Geometry check sheet. Reference: the model listing, model coordinates, mm. A direction names the side the tool comes from. Coordinates: 2 decimals unless noted, no trailing zeros. Write each loop counter-clockwise with the first axis right and the second up, starting at its lowest first coordinate (ties: lowest second). Pieces come first, ordered by that corner, then holes. Notation, with made-up numbers: (64, 69) -> (111, 69) arc R31 cw to (111, 107) -> close; hole circle Ø8 at (19.25, -14.75). An arc over 180 degrees is marked (long way). Put each result on its own line as item: value. Start each with the question number.
from build123d import *

# Parameters (mm, degrees)
EXTRUDE_1_DEPTH     = 40
SKETCH_4_W          = 8
SKETCH_4_H          = 8
EXTRUDE_2_DEPTH     = 8
SKETCH_5_R          = 1.98
CUT_EXTRUDE_2_DEPTH = 8
FILLET_1_R          = 10
FILLET_2_R          = 10
SKETCH_6_W          = 8
SKETCH_6_H          = 8
EXTRUDE_3_DEPTH     = 8
SKETCH_7_R          = 1.98
CUT_EXTRUDE_3_DEPTH = 8
FILLET_3_R          = 10
FILLET_4_R          = 10


with BuildPart() as part:
    # 草图2 → 凸台-拉伸1 (new body)
    with BuildSketch(Plane(origin=(0, 0, 0), x_dir=(0, 0, -1), z_dir=(1, 0, 0))):
        Polygon((0, 0), (0, -42), (-25.455844123, -67.455844123), (-27.930717857, -64.980970389), (-3.5, -40.550252532), (-3.5, 0), align=None)
    extrude(amount=EXTRUDE_1_DEPTH)

    # 草图4 → 凸台-拉伸2 (add)
    with BuildSketch(Plane.ZY):
        with Locations((1.75, -4)):
            Rectangle(SKETCH_4_W, SKETCH_4_H)
    extrude(amount=EXTRUDE_2_DEPTH)

    # 草图5 → 切除-拉伸2 (cut)
    with BuildSketch(Plane(origin=(0, 0, 0), x_dir=(1, 0, 0), z_dir=(0, 1, 0))):
        with Locations(Location((-4, -1.75, 0), (0, 0, 270))):
            Circle(SKETCH_5_R)
    extrude(amount=-CUT_EXTRUDE_2_DEPTH, mode=Mode.SUBTRACT)

    # 圆角1
    # the kernel refuses this fillet: 10 mm, written as the material it adds along each edge
    with BuildSketch(Plane(origin=(0, 0, 0), x_dir=(1, 0, 0), z_dir=(0, -1, 0))) as fillet_1_piece_1:
        with BuildLine():
            CenterArc((6.31961233, -10), FILLET_1_R, 90, 39.194967426)
            Line((0, -2.25), (0, 0))
            Line((0, 0), (6.31961233, 0))
        make_face()
    extrude(amount=8)

    # 圆角2
    # the kernel refuses this fillet: 10 mm, written as the material it adds along each edge
    with BuildSketch(Plane(origin=(0, -8, 3.5), x_dir=(1, 0, 0), z_dir=(0, 1, 0))) as fillet_2_piece_1:
        with BuildLine():
            CenterArc((6.31961233, -10), FILLET_2_R, 90, 39.194967426)
            Line((0, -2.25), (0, 0))
            Line((0, 0), (6.31961233, 0))
        make_face()
    extrude(amount=8)

    # 草图6 → 凸台-拉伸3 (add)
    with BuildSketch(Plane(origin=(40, 0, 0), x_dir=(0, 0, -1), z_dir=(1, 0, 0))):
        with Locations((-1.75, -4)):
            Rectangle(SKETCH_6_W, SKETCH_6_H)
    extrude(amount=EXTRUDE_3_DEPTH)

    # 草图7 → 切除-拉伸3 (cut)
    with BuildSketch(Plane(origin=(0, 0, 0), x_dir=(1, 0, 0), z_dir=(0, 1, 0))):
        with Locations(Location((44, -1.75, 0), (0, 0, 270))):
            Circle(SKETCH_7_R)
    extrude(amount=-CUT_EXTRUDE_3_DEPTH, mode=Mode.SUBTRACT)

    # 圆角3
    # the kernel refuses this fillet: 10 mm, written as the material it adds along each edge
    with BuildSketch(Plane(origin=(40, 0, 0), x_dir=(-1, 0, 0), z_dir=(0, -1, 0))) as fillet_3_piece_1:
        with BuildLine():
            CenterArc((6.31961233, 10), FILLET_3_R, 230.805032574, 39.194967426)
            Line((0, 2.25), (0, 0))
            Line((0, 0), (6.31961233, 0))
        make_face()
    extrude(amount=8)

    # 圆角4
    # the kernel refuses this fillet: 10 mm, written as the material it adds along each edge
    with BuildSketch(Plane(origin=(40, -8, 3.5), x_dir=(-1, 0, 0), z_dir=(0, 1, 0))) as fillet_4_piece_1:
        with BuildLine():
            CenterArc((6.31961233, 10), FILLET_4_R, 230.805032574, 39.194967426)
            Line((0, 2.25), (0, 0))
            Line((0, 0), (6.31961233, 0))
        make_face()
    extrude(amount=8)


solid = part.part
Item 1: Section check C-C, the plane y = -31. Enter the section's corners in (x, z), and give its area (3 significant figures).
Item 2: Section check D-D, the plane x = 21.5. Enter the section's corners in (y, z), and give its area (3 significant figures).
Item 3: Scan lines: line 1 along X through (y, z) = (-3.75, 1.75); line 2 along Z through (x, y) = (6, -31); line 3 along Y through (x, z) = (-1.5, 5). Record each from-to range of solid material in increasing order. Write a range as [from, to].
Item 4: Section check A-A, the plane z = 1.75. Enter the section's corners in (x, y), and give its area (3 significant figures).
Item 5: Access from +Z, -Z, +X, -X, +Y, -Y to the whole of each face (thin tool, end or side, straight path). Record for faces 1 (the flat face through (20, -21, 0)), 2 (the flat face through (20, -21, 3.5)), 3 (the cylindrical face through (37.08, -3.944, -0.595)), 4 (the flat face through (0, -42, 4.6)), 5 (the cylindrical face through (3.011, -4.056, 4.063)).
Item 6: Mould release check, pull along Z, two halves, no side actions. Record for faces 6 (the cylindrical face through (45.963, -3.944, 1.492)), 7 (the flat face through (19.72, -66.236, 26.676)), 8 (the flat face through (40, -42, 4.6)): released by +Z, released by -Z, zero draft, split by the parting line, or undercut.
Item 7: Go/stop test with flat-tipped pins: P1, Ø12, axis at x = 26.5, y = -28, coming from the -Z side; P2, Ø1.5, axis at x = 5, y = -53, coming from the -Z side; P3, Ø10, axis at x = -1, y = -10, coming from the +Z side; P4, Ø8.5, axis at y = -26, z = 9, coming from the -X side. Record where each tip stops, or that it passes through.
Item 8: Section check B-B, the plane x = -4. Enter the section's corners in (y, z).
From the geometry:
1. outline: (0, 0) -> (40, 0) -> (40, 3.5) -> (0, 3.5) -> close
1. area: 140 mm²
2. outline: (-67.46, 25.46) -> (-42, 0) -> (0, 0) -> (0, 3.5) -> (-40.55, 3.5) -> (-64.98, 27.93) -> close
2. area: 268 mm²
3. line 1: [-8, -5.98], [-2.02, 42.02], [45.98, 48]
3. line 2: [0, 3.5]
3. line 3: [-8, 0]
4. outline: (-8, -8) -> (-5.98, -8) -> (-5.98, 0) -> (-8, 0) -> close; (-2.02, -8) -> (0, -8) -> (0, -43.75) -> (40, -43.75) -> (40, -8) -> (42.02, -8) -> (42.02, 0) -> (-2.02, 0) -> close; (45.98, -8) -> (48, -8) -> (48, 0) -> (45.98, 0) -> close
4. area: 1,810 mm²
5. face 1: -Z, -Y
5. face 2: +Z
5. face 3: -Z, +Y, -Y
5. face 4: +Z, -Z, -X, -Y
5. face 5: +Z, +Y
6. face 6: undercut
6. face 7: released by +Z
6. face 8: zero draft
7. P1: z = 0
7. P2: z = 10.25
7. P3: z = 5.75
7. P4: through
8. outline: (-8, -2.25) -> (0, -2.25) -> (0, -0.23) -> (-8, -0.23) -> close; (-8, 3.73) -> (0, 3.73) -> (0, 5.75) -> (-8, 5.75) -> close
